Autodesk Fusion 360 part; units mm, degrees
sketch "Sketch1" plane through (0, 0, 0) normal (1, 0, 0) x (0, 1, 0)
sketch "Sketch2" plane through (0, 0, 0) normal (0, 1, 0) x (1, 0, 0)
sketch "Sketch3" plane through (0, 0, 0) normal (0, 0, 1) x (1, 0, 0)
  line L0 (-89.6492, -40) -> (80, -40)
  line L1 (80, -40) -> (80, 40)
  line L2 (80, 40) -> (-89.6492, 40)
  line L3 (-89.6492, 40) -> (-89.6492, 30)
  line L4 (-89.6492, -40) -> (-89.6492, -30)
  line L5 (-89.6492, -40) -> (-79.6492, -40)
  line L6 (-79.6492, 27.5) -> (-79.6492, -27.5)
  line L7 (-79.6492, 27.5) -> (-89.6492, 30)
  line L8 (-89.6492, -30) -> (-79.6492, -27.5)
extrude "Extrude1" add sketch "Sketch3" along normal blind 2.5
sketch "Sketch4" plane through (0, 0, 2.5) normal (0, 0, 1) x (-1, 0, 0)
  line L0 (89.6492, 40) -> (-80, 40)
  line L1 (-80, 40) -> (-80, -40)
  line L2 (-80, -40) -> (89.6492, -40)
  line L3 (89.6492, -40) -> (89.6492, -30)
  line L4 (89.6492, -30) -> (79.6492, -27.5)
  line L5 (79.6492, -27.5) -> (79.6492, 27.5)
  line L6 (79.6492, 27.5) -> (89.6492, 30)
  line L7 (89.6492, 30) -> (89.6492, 40)
  line L8 (89.6492, -40) -> (-80, -40)
  line L9 (-80, -40) -> (-80, 40)
  line L10 (89.6492, 40) -> (-80, 40)
  line L11 (89.6492, 30) -> (89.6492, 40)
  line L12 (89.6492, 30) -> (79.6492, 27.5)
  line L13 (79.6492, 27.5) -> (79.6492, -27.5)
  line L14 (79.6492, -27.5) -> (89.6492, -30)
  line L15 (89.6492, -40) -> (89.6492, -30)
  line L16 (89.6492, -40) -> (89.6492, -38.5)
  line L17 (88.1492, -38.5) -> (-78.5, -38.5)
  line L18 (-80, -40) -> (-78.5, -40)
  line L19 (-78.5, -38.5) -> (-78.5, 38.5)
  line L20 (-80, 40) -> (-80, 38.5)
  line L21 (-78.5, 38.5) -> (88.1492, 38.5)
  line L22 (89.6492, 40) -> (88.1492, 40)
  line L23 (88.1492, 38.5) -> (88.1492, 31)
  line L24 (89.6492, 30) -> (89.6492, 31.375)
  line L25 (88.1492, 31) -> (78.1492, 28.5)
  line L26 (78.1492, -28.4841) -> (78.1492, 28.5)
  line L27 (89.6492, -40) -> (88.1492, -40)
  line L28 (88.1492, -31.1066) -> (88.1492, -38.5)
  line L29 (89.6492, -30) -> (89.6492, -31.5)
  line L30 (88.1492, -31.1066) -> (78.1492, -28.4841)
  dimension "d9" = 1.5
  dimension "d11" = 1.5
Read the model definition and answer for the solid it produces. Units are mm, in the model's axes. Give positions to 0.01 mm unless a question says otherwise; leave off trailing zeros. Write each loop counter-clockwise with the first axis right and the second up, starting at its lowest first coordinate (ties: lowest second). Pieces come first, ordered by that corner, then holes. Notation, with made-up numbers: M -39.75,20 L 3.25,20 A13 cw 3.25,35 Z; hole C 83,51.25 d8. An arc over 180 degrees is marked long. Put each result on its own line as item: value. Start each with the question number.
1. This flat-tipped pin is pushed along its axis until it touches: pin 1 Ø0.8 at (y, z) = (4, 1) entering from -X. Where does it stop, or does it pass through?
2. Consider line 1 along X through (y, z) = (-25.5, 2.1); line 2 along Y through (x, z) = (-82, 1.75). Determine where each line is inside the solid, lowest interval first.
3. The part is cut by section B-B, the plane y = 1.5. Give the vertices of the cut face in (x, z), and give its area (3 significant figures).
4. The part is cut by section A-A, the plane z = 1.6. Give the vertices of the cut face in (x, y), and give its area (3 significant figures).
Final values:
1. pin 1: stops at x = -79.65
2. line 1: x = -79.65 to 80
2. line 2: y = -40 to -28.09, 28.09 to 40
3. outline: M -79.65,0 L 80,0 L 80,2.5 L -79.65,2.5 Z
3. area: 399 mm²
4. outline: M -89.65,-40 L 80,-40 L 80,40 L -89.65,40 L -89.65,30 L -79.65,27.5 L -79.65,-27.5 L -89.65,-30 Z
4. area: 13,000 mm²
